Could you check a few things on this drawing? It's one solid part, dimensions in mm from its lowest x, y, z. Coordinates: 2 decimals unless noted, no trailing zeros. Order: outer loops, then holes, each group sorted by start corner. A loop starts at its lowest first (then second) coordinate and runs counter-clockwise, first axis right, second up. Notation, with made-up numbers: (53.5, 72) - (81.5, 72) arc R6 ccw to (81.5, 76) - close; hole circle Ø11 at (60, -19.5). An arc over 180 degrees is marked (long way). Return JSON: item names as keys, results as strings. Group by question number.
1) If we mould it in two halves opening along Y, with no side actions, what happens to the marked faces 1 and 2? For each: pulls with the +Y half, pulls with the -Y half, needs draft (parallel to the pull), parting line crosses it, or undercut.
2) Imagine slicing it at A-A (x = 53). Write out the boundary of the cut face in (y, z) (1 decimal).
3) If I drill on line 1 along Z through (x, y) = (51, 49); line 2 along X through (y, z) = (44.5, 7.25) (1 decimal); line 3 along X through (y, z) = (25.5, 7.75) (1 decimal), over which ranges is the centre line in solid material (lowest first)?
4) Imagine slicing it at B-B (y = 30). Write out the boundary of the cut face in (x, z) (1 decimal).
5) Imagine slicing it at D-D (x = 37). Write out the boundary of the cut face in (y, z) (1 decimal).
6) For pin 1 Ø3 at (x, z) = (11.5, 1.5) entering from +Y; pin 2 Ø3 at (x, z) = (21.5, 1.5) entering from -Y; pin 3 Ø3 at (x, y) = (22, 50) entering from +Z, each with a flat end and sliding along its axis, tell me the tip position at first contact or that it passes through.
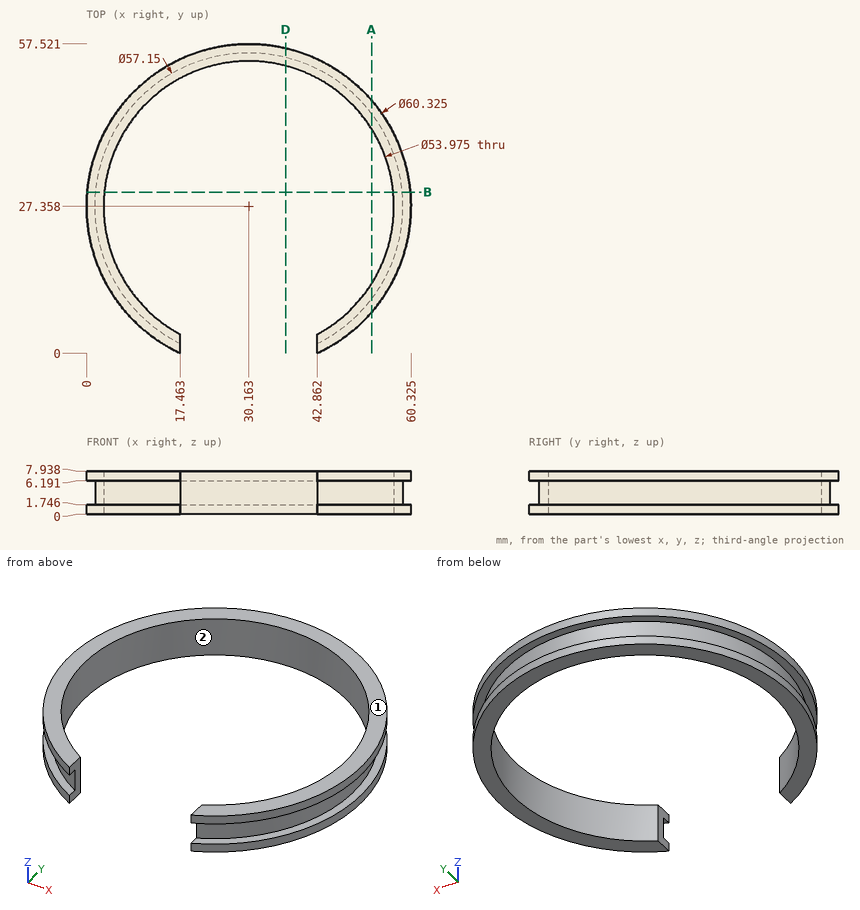
Calculated:
{
 "1": {"face 1": "needs draft", "face 2": "undercut"},
 "2": {"outline": "(7.7, 0) - (13, 0) - (13, 7.9) - (7.7, 7.9) - (7.7, 6.2) - (10.2, 6.2) - (10.2, 1.7) - (7.7, 1.7) - close; (41.7, 0) - (47.1, 0) - (47.1, 1.7) - (44.5, 1.7) - (44.5, 6.2) - (47.1, 6.2) - (47.1, 7.9) - (41.7, 7.9) - close"},
 "3": {"line 1": "0 to 1.75, 6.19 to 7.94", "line 2": "5.3 to 9.3, 51 to 55", "line 3": "0.1 to 3.2, 57.1 to 60.3"},
 "4": {"outline": "(0.1, 0) - (3.3, 0) - (3.3, 7.9) - (0.1, 7.9) - (0.1, 6.2) - (1.7, 6.2) - (1.7, 1.7) - (0.1, 1.7) - close; (57, 0) - (60.2, 0) - (60.2, 1.7) - (58.6, 1.7) - (58.6, 6.2) - (60.2, 6.2) - (60.2, 7.9) - (57, 7.9) - close"},
 "5": {"outline": "(53.5, 0) - (56.7, 0) - (56.7, 1.7) - (55.1, 1.7) - (55.1, 6.2) - (56.7, 6.2) - (56.7, 7.9) - (53.5, 7.9) - close"},
 "6": {"pin 1": "y = 52.16", "pin 2": "y = 52.36", "pin 3": "through"}
}
